For this review, take the finished solid that the model builds, in its own axes (mm). A direction names the side the tool comes from. Give positions to 0.01 mm unless a question says otherwise; leave off trailing zeros. Loops run counter-clockwise (first coordinate to the right, second up) from the corner with the lowest first, then second, coordinate; pieces in that order, holes last. Notation, with made-up numbers: (37.5, 24) - (65.5, 24) arc R12 ccw to (65.5, 42) - close; hole circle Ø8 at (-17, 45). An arc over 180 degrees is marked (long way). Put each result on its own line as item: value.
from build123d import *

# Parameters (mm, degrees)
SKETCH1_W               = 110
SKETCH1_H               = 189
BOSS_EXTRUDE1_DEPTH     = 4
SKETCH3_W               = 10
SKETCH3_H               = 162
BOSS_EXTRUDE2_DEPTH     = 3
CUT_EXTRUDE1_DEPTH      = 5
CUT_EXTRUDE1_DEPTH_BACK = 146
SKETCH2_R               = 2.5
SKETCH2_R_2             = 1.12
SKETCH4_R               = 12.7
CUT_EXTRUDE2_DEPTH      = 5


with BuildPart() as part:
    # Sketch1 → Boss-Extrude1 (new body)
    with BuildSketch(Plane.XY):
        with Locations((55, 94.5)):
            Rectangle(SKETCH1_W, SKETCH1_H)
    extrude(amount=BOSS_EXTRUDE1_DEPTH)

    # Sketch3 → Boss-Extrude2 (add)
    with BuildSketch(Plane.XY.offset(4)):
        with Locations((55, 97)):
            Rectangle(SKETCH3_W, SKETCH3_H)
        with Locations((20, 97)):
            Rectangle(SKETCH3_W, SKETCH3_H)
        with Locations((90, 97)):
            Rectangle(SKETCH3_W, SKETCH3_H)
    extrude(amount=BOSS_EXTRUDE2_DEPTH)

    # Sketch2 → Cut-Extrude1 (cut, two sides: drawn at the far end of the back side and taken through both)
    with BuildSketch(Plane.XY.offset(4).offset(-CUT_EXTRUDE1_DEPTH_BACK)):
        with Locations(Location((20, 12, 0), (0, 0, 180))):
            Circle(SKETCH2_R)
        with Locations(Location((90, 12, 0), (0, 0, 180))):
            Circle(SKETCH2_R)
        with Locations(Location((18.86, 25.4, 0), (0, 0, 180))):
            Circle(SKETCH2_R)
        with Locations(Location((91.14, 25.4, 0), (0, 0, 180))):
            Circle(SKETCH2_R)
        with Locations(Location((20, 182, 0), (0, 0, 180))):
            Circle(SKETCH2_R)
        with Locations(Location((90, 182, 0), (0, 0, 180))):
            Circle(SKETCH2_R)
        with Locations(Location((70, 134, 0), (0, 0, 180))):
            Circle(SKETCH2_R_2)
        with Locations(Location((90, 134, 0), (0, 0, 180))):
            Circle(SKETCH2_R_2)
        with Locations(Location((90, 114, 0), (0, 0, 180))):
            Circle(SKETCH2_R_2)
        with Locations(Location((70, 114, 0), (0, 0, 180))):
            Circle(SKETCH2_R_2)
    extrude(amount=CUT_EXTRUDE1_DEPTH + CUT_EXTRUDE1_DEPTH_BACK, mode=Mode.SUBTRACT)

    # Sketch4 → Cut-Extrude2 (cut)
    with BuildSketch(Plane(origin=(0, 0, 0), x_dir=(-1, 0, 0), z_dir=(0, 0, -1))):
        with Locations((-55, 164)):
            Circle(SKETCH4_R)
    extrude(amount=-CUT_EXTRUDE2_DEPTH, mode=Mode.SUBTRACT)


solid = part.part
1) Draft analysis for pull direction X (two halves, no side actions). For faces 3 (the face through (110, 93, 2)), 4 (the face through (42, 96, 4)), 5 (the face through (55, 98, 7)), 6 (the face through (0, 93, 2)), state which applies: pulls with the +X half, pulls with the -X half, needs draft (parallel to the pull), parting line crosses it, or undercut.
Geometry check:
face 3: pulls with the +X half
face 4: undercut
face 5: needs draft
face 6: pulls with the -X half
2) Take a section at A-A on y = 12. State the section outline as (x, z) points, and give its area (3 significant figures).
Geometry check:
outline: (0, 0) - (17.5, 0) - (17.5, 4) - (0, 4) - close; (22.5, 0) - (87.5, 0) - (87.5, 4) - (22.5, 4) - close; (92.5, 0) - (110, 0) - (110, 4) - (92.5, 4) - close
area: 400 mm²
3) For faces 1 (the face through (16.55, 26.36, 3.45)), 2 (the face through (55, 164, 5)), list the 3-axis set-ups (+Z, -Z, +X, -X, +Y, -Y) from which the entire face can be reached by the end or side of a thin tool; tool diameter is ignored.
Geometry check:
face 1: +Z, -Z
face 2: -Z
4) Take a section at B-B on z = 2.25. State how many separate pieces and enclosed holes the cut face has, and give its area (3 significant figures).
Geometry check:
separate pieces: 1
enclosed holes: 11
area: 20,100 mm²
5) Wall thickness on line 1 (X direction, y = 182, z = 2); line 2 (X direction, y = 140, z = 5); line 3 (X direction, y = 114, z = 5): over which ranges is each line inside the solid? List them lowest first.
Geometry check:
line 1: x = 0 to 17.5, 22.5 to 87.5, 92.5 to 110
line 2: x = 15 to 25, 50 to 60, 85 to 95
line 3: x = 15 to 25, 50 to 60, 85 to 88.88, 91.12 to 95
6) Insertion check: pin 1 Ø2.5 at (y, z) = (115, 6) entering from +X; pin 2 Ø0.9 at (y, z) = (103.5, 5.5) entering from -X; pin 3 Ø1.5 at (x, z) = (90, 5.5) entering from +Y; pin 4 Ø1.3 at (x, y) = (90, 114) entering from +Z. Each pin has a flat end and moves straight along its axis. Give the tip position at first contact, or say it passes through.
Geometry check:
pin 1: stops at x = 95
pin 2: stops at x = 15
pin 3: stops at y = 178
pin 4: passes through
7) Take a section at C-C on y = 88. State the section outline as (x, z) points, and give its area (3 significant figures).
Geometry check:
outline: (0, 0) - (110, 0) - (110, 4) - (95, 4) - (95, 7) - (85, 7) - (85, 4) - (60, 4) - (60, 7) - (50, 7) - (50, 4) - (25, 4) - (25, 7) - (15, 7) - (15, 4) - (0, 4) - close
area: 530 mm²
8) Take a section at D-D on x = 55. State the section outline as (y, z) points.
Geometry check:
outline: (0, 0) - (151.3, 0) - (151.3, 5) - (176.7, 5) - (176.7, 0) - (189, 0) - (189, 4) - (178, 4) - (178, 7) - (16, 7) - (16, 4) - (0, 4) - close
